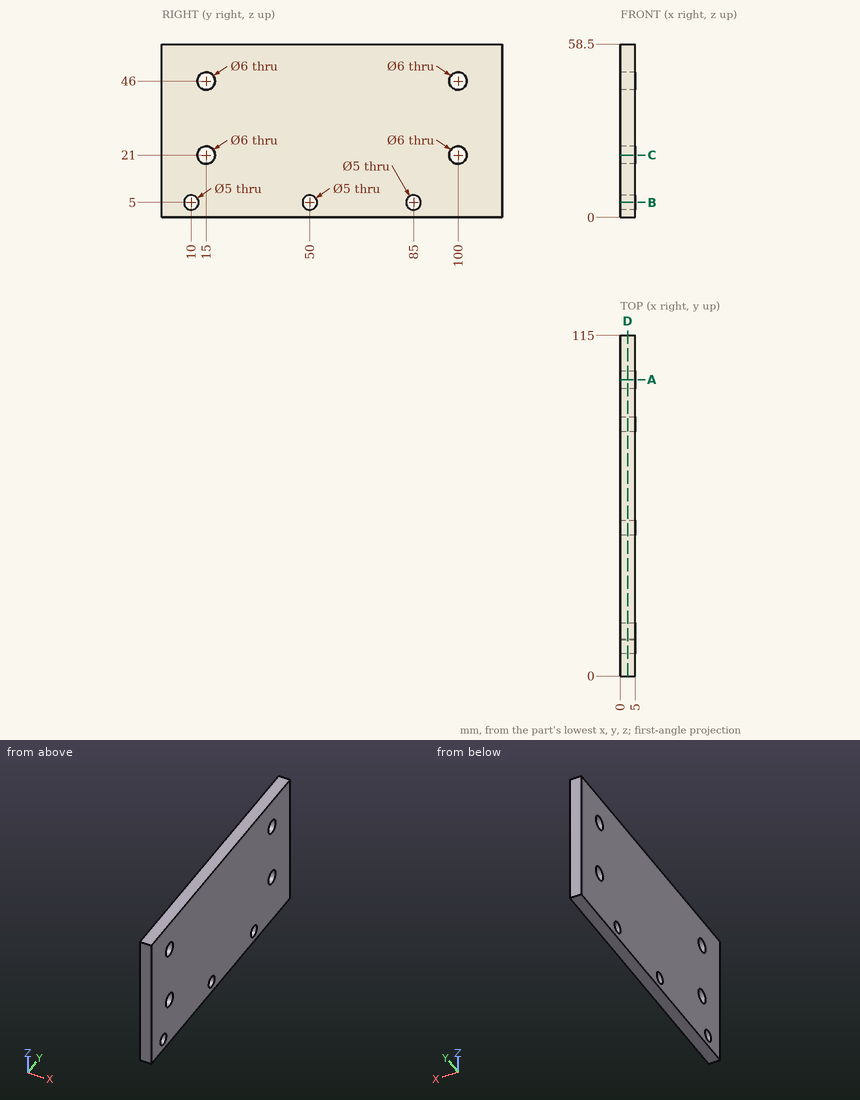
Study the drawing (mm; zero at the part's minimum x, y, z) and answer. Round coordinates to 2 decimals unless told otherwise and drop trailing zeros. Loops run counter-clockwise (first coordinate to the right, second up) from the corner with the lowest first, then second, coordinate; pieces in that order, holes last.
Q1. Section B-B, the plane z = 5 is taken. Determine the outline of the cut face in (x, y).
Q2. Find the intervals of material crossed by line 1 (Z direction, x = 1.75, y = 100); line 2 (Y direction, x = 1.75, z = 46); line 3 (Y direction, x = 1.6, z = 48.5), in increasing order.
Q3. Section D-D, the plane x = 2.4 is taken. Determine the outline of the cut face in (y, z), then the cut area to 3 significant figures.
Q4. Section C-C, the plane z = 21 is taken. Determine the outline of the cut face in (x, y).
Q5. Given pin 1 Ø4 at (y, z) = (10, 5) entering from +X, flat-ended and moving along its own axis, determine where the tip first touches the part or whether it passes through.
Q6. Section A-A, the plane y = 100 is taken. Determine the outline of the cut face in (x, z), then the cut area to 4 significant figures.
Completed:
1. outline: (0, 0) - (5, 0) - (5, 7.5) - (0, 7.5) - close; (0, 12.5) - (5, 12.5) - (5, 47.5) - (0, 47.5) - close; (0, 52.5) - (5, 52.5) - (5, 82.5) - (0, 82.5) - close; (0, 87.5) - (5, 87.5) - (5, 115) - (0, 115) - close
2. line 1: z = 0 to 18, 24 to 43, 49 to 58.5
2. line 2: y = 0 to 12, 18 to 97, 103 to 115
2. line 3: y = 0 to 13.34, 16.66 to 98.34, 101.66 to 115
3. outline: (0, 0) - (115, 0) - (115, 58.5) - (0, 58.5) - close; hole circle Ø5 at (10, 5); hole circle Ø6 at (15, 21); hole circle Ø6 at (15, 46); hole circle Ø5 at (50, 5); hole circle Ø5 at (85, 5); hole circle Ø6 at (100, 21); hole circle Ø6 at (100, 46)
3. area: 6,560 mm2
4. outline: (0, 0) - (5, 0) - (5, 12) - (0, 12) - close; (0, 18) - (5, 18) - (5, 97) - (0, 97) - close; (0, 103) - (5, 103) - (5, 115) - (0, 115) - close
5. pin 1: passes through
6. outline: (0, 0) - (5, 0) - (5, 18) - (0, 18) - close; (0, 24) - (5, 24) - (5, 43) - (0, 43) - close; (0, 49) - (5, 49) - (5, 58.5) - (0, 58.5) - close
6. area: 232.5 mm2
